Part model, mm, in its own coordinate system. A direction names the side the tool comes from. Round coordinates to 2 decimals unless told otherwise and drop trailing zeros. Write each loop counter-clockwise with the first axis right and the second up, starting at its lowest first coordinate (ties: lowest second). Pieces come first, ordered by that corner, then holes. Notation, with made-up numbers: M 54.5,-3 L 65.5,-3 A27 cw 65.5,25 Z; hole C 50,-28.75 d10. An arc over 180 degrees is marked long. Answer as a JSON object with one key per item and string values. Group by question number.
1. Drop flat-ended pins along their axis: pin 1 (3 mm diameter, centred on y = -20, z = 10, fed in from -X); pin 2 (2.5 mm diameter, centred on x = -38.5, y = -10, fed in from -Z); pin 3 (1.5 mm diameter, centred on y = -26.5, z = 16.5, fed in from -X); pin 4 (8.5 mm diameter, centred on x = -37, y = -26.5, fed in from -Z). Give the stop position or say it passes through.
2. Two-plate mould, pull along Z, no slides. Class faces 4 (the face through (-41.246, -39.26, 17.465)), 5 (the face through (-28.535, -12.197, 12.395)), 6 (the face through (-29, -20, 2)): +Z half, -Z half, draft (parallel to the pull), parting line (faces both ways), or undercut.
3. Drill centre lines: line 1 (Y direction, x = -27.7, z = 10); line 2 (X direction, y = -5, z = 18.7); line 3 (Z direction, x = -32, y = -21). Where is each one in solid material? Low to high. Write a range as from..to.
4. Which spindle directions (+Z, -Z, +X, -X, +Y, -Y) get a long thin tool onto all of the face, cutting with end or side? Do faces 1 (the face through (-41, -20, 18)), 2 (the face through (-30, -40, 12)), 3 (the face through (-31, -20, 8)). Say none if no direction does.
5. Band-saw the part on C-C, the plane x = -30. Write the cut outline in (y, z).
6. Band-saw the part on B-B, the plane y = -10. Write the cut outline in (x, z).
7. Band-saw the part on D-D, the plane y = -25. Write the cut outline in (x, z).
8. Band-saw the part on A-A, the plane z = 10. Write the cut outline in (x, y), plus the area to 3 significant figures.
from build123d import *

# Parameters (mm, degrees)
SKETCH008_W     = 20
SKETCH008_H     = 40
SKETCH008_R     = 2.75
SKETCH008_R_2   = 1.3
PAD004_DEPTH    = 5
SKETCH009_W     = 5
SKETCH009_H     = 40
PAD005_DEPTH    = 15
SKETCH010_R     = 1.5
POCKET004_DEPTH = 5.001
SKETCH011_W     = 37
SKETCH011_H     = 6
POCKET005_DEPTH = 3
CHAMFER007_SIZE = 2
CHAMFER008_SIZE = 4
CHAMFER009_SIZE = 5
POCKET007_DEPTH = 5
SKETCH018_R     = 3.25
POCKET011_DEPTH = 7
SKETCH019_W     = 2
SKETCH019_H     = 2
POCKET012_DEPTH = 40.001


with BuildPart() as part:
    # Sketch008 (on DatumPlane) → Pad004 (new body)
    with BuildSketch(Plane(origin=(-5, 0, 20), x_dir=(0, 0, -1), z_dir=(-1, 0, 0))):
        with Locations((10, 20)):
            Rectangle(SKETCH008_W, SKETCH008_H)
        with Locations((10, 30)):
            Circle(SKETCH008_R, mode=Mode.SUBTRACT)
        with Locations((10, 10)):
            Circle(SKETCH008_R, mode=Mode.SUBTRACT)
        with Locations((10, 20)):
            Circle(SKETCH008_R_2, mode=Mode.SUBTRACT)
    extrude(amount=PAD004_DEPTH)

    # Sketch009 (on Face9 of Pad004) → Pad005 (join)
    with BuildSketch(Plane(origin=(-10, 0, 20), x_dir=(0, 0, -1), z_dir=(-1, 0, 0))):
        with Locations((2.5, 20)):
            Rectangle(SKETCH009_W, SKETCH009_H)
    extrude(amount=PAD005_DEPTH)

    # Sketch010 (on Face7 of Pad005) → Pocket004 (cut, through all)
    with BuildSketch(Plane(origin=(-5, 0, 15), x_dir=(0, -1, 0), z_dir=(0, 0, -1))):
        with Locations((5, 12.5)):
            Circle(SKETCH010_R)
        with Locations((10, 12.5)):
            Circle(SKETCH010_R)
        with Locations((15, 12.5)):
            Circle(SKETCH010_R)
        with Locations((20, 12.5)):
            Circle(SKETCH010_R)
        with Locations((25, 12.5)):
            Circle(SKETCH010_R)
        with Locations((30, 12.5)):
            Circle(SKETCH010_R)
        with Locations((35, 12.5)):
            Circle(SKETCH010_R)
    extrude(amount=-POCKET004_DEPTH, mode=Mode.SUBTRACT)

    # Sketch011 (on Face18 of Pocket004) → Pocket005 (cut)
    with BuildSketch(Plane(origin=(-5, 0, 15), x_dir=(0, -1, 0), z_dir=(0, 0, -1))):
        with Locations((20, 12.5)):
            Rectangle(SKETCH011_W, SKETCH011_H)
    extrude(amount=-POCKET005_DEPTH, mode=Mode.SUBTRACT)

    # Chamfer007
    chamfer007_edges = [part.edges().sort_by_distance(p)[0] for p in [
        (-10, -20, 15),
    ]]
    chamfer(chamfer007_edges, length=CHAMFER007_SIZE)

    # Chamfer008
    chamfer008_edges = [part.edges().sort_by_distance(p)[0] for p in [
        (-10, -20, 0),
    ]]
    chamfer(chamfer008_edges, length=CHAMFER008_SIZE)

    # Chamfer009
    chamfer009_edges = [part.edges().sort_by_distance(p)[0] for p in [
        (-25, 0, 17.5),
        (-25, -40, 17.5),
    ]]
    chamfer(chamfer009_edges, length=CHAMFER009_SIZE)

    # Sketch012 (on Face2 of Chamfer009) → Pocket007 (cut)
    with BuildSketch(Plane(origin=(-5, 0, 15), x_dir=(0, -1, 0), z_dir=(0, 0, -1))):
        Polygon((0, 15), (5, 20), (35, 20), (40, 15), (38.5, 15.5), (1.5, 15.5), align=None)
    extrude(amount=-POCKET007_DEPTH, mode=Mode.SUBTRACT)

    # Sketch018 (on Face6 of Pocket007) → Pocket011 (cut)
    with BuildSketch(Plane(origin=(-10, 0, 20), x_dir=(0, 0, -1), z_dir=(-1, 0, 0))):
        with Locations((10, 30)):
            Circle(SKETCH018_R)
        with Locations((10, 10)):
            Circle(SKETCH018_R)
    extrude(amount=-POCKET011_DEPTH, mode=Mode.SUBTRACT)

    # Sketch019 (on Face1 of Pocket011) → Pocket012 (cut, through all)
    with BuildSketch(Plane(origin=(-5, 0, 20), x_dir=(0, 0, -1), z_dir=(0, 1, 0))):
        with Locations((6, 6)):
            Rectangle(SKETCH019_W, SKETCH019_H)
    extrude(amount=-POCKET012_DEPTH, mode=Mode.SUBTRACT)


with BuildPart() as part_1:
    # Body003 placement: moved
    add(part.part.moved(Location((-21, 0, 0))))


solid = part_1.part
Worked answers:
{
 "1": {"pin 1": "stops at x = -31", "pin 2": "passes through", "pin 3": "stops at x = -35.5", "pin 4": "stops at z = 15"},
 "2": {"face 4": "draft", "face 5": "undercut", "face 6": "-Z half"},
 "3": {"line 1": "y = -40..-33.25, -26.75..-21.3, -18.7..-13.25, -6.75..0", "line 2": "x = -41.5..-40, -37..-26", "line 3": "z = 15..20"},
 "4": {"face 1": "-Z, -X", "face 2": "+Z, -Z, +X, -X, -Y", "face 3": "-Z, -X, +Y, -Y"},
 "5": {"outline": "M -40,3 L 0,3 L 0,20 L -40,20 Z; hole C -30,10 d6.5; hole C -20,10 d2.6; hole C -10,10 d6.5"},
 "6": {"outline": "M -41.5,18 L -40,18 L -40,20 L -41.5,20 Z; M -37,18 L -35.5,18 L -35.5,15 L -31,15 L -31,13.25 L -26,13.25 L -26,20 L -37,20 Z; M -31,4 L -27,0 L -26,0 L -26,6.75 L -31,6.75 Z"},
 "7": {"outline": "M -41.5,18 L -40,18 L -40,20 L -41.5,20 Z; M -37,18 L -35.5,18 L -35.5,15 L -31,15 L -31,4 L -27,0 L -26,0 L -26,20 L -37,20 Z"},
 "8": {"outline": "M -31,-40 L -26,-40 L -26,-33.25 L -31,-33.25 Z; M -31,-26.75 L -26,-26.75 L -26,-21.3 L -31,-21.3 Z; M -31,-18.7 L -26,-18.7 L -26,-13.25 L -31,-13.25 Z; M -31,-6.75 L -26,-6.75 L -26,0 L -31,0 Z", "area": "122 mm^2"}
}
